Autodesk Inventor part; units mm, degrees
ref_plane "YZ Plane" through (0, 0, 0) normal (1, 0, 0) x (0, 1, 0)
ref_plane "XZ Plane" through (0, 0, 0) normal (0, 1, 0) x (-1, 0, 0)
ref_plane "XY Plane" through (0, 0, 0) normal (0, 0, 1) x (1, 0, 0)
sketch "Sketch1" plane through (0, 0, 0) normal (0, 0, 1) x (1, 0, 0)
  circle A0 centre (0, 0) radius 9.53
  dimension "d0" = 19.06
extrude "Extrusion1" add sketch "Sketch1" against normal blind 20.62
sketch "Sketch2" plane through (0, 0, 0) normal (0, 0, 1) x (1, 0, 0)
  circle A0 centre (0, 0) radius 5.795
  dimension "d3" = 11.59
extrude "Extrusion2" add sketch "Sketch2" along normal blind 6.35
sketch "Sketch3" plane through (0, 0, 6.35) normal (0, 0, 1) x (1, 0, 0)
  circle A0 centre (0, 0) radius 7
  dimension "d6" = 14
extrude "Extrusion3" add sketch "Sketch3" along normal blind 100
sketch "Sketch4" plane through (0, 0, 106.35) normal (0, 0, 1) x (1, 0, 0)
  circle A0 centre (0, 0) radius 7
  circle A1 centre (0, 0) radius 7
  circle A2 centre (0, 0) radius 7
  circle A3 centre (0, 0) radius 5.795
extrude "Extrusion4" add sketch "Sketch4" along normal blind 22.1 contours A3
sketch "Sketch5" plane through (0, 0, 128.45) normal (0, 0, 1) x (1, 0, 0)
  circle A0 centre (0, 0) radius 4.76
  dimension "d11" = 9.52
extrude "Extrusion5" add sketch "Sketch5" along normal blind 3.33
sketch "Sketch6" plane through (0, 0, 131.78) normal (0, 0, 1) x (1, 0, 0)
  circle A0 centre (0, 0) radius 5.795
extrude "Extrusion6" add sketch "Sketch6" along normal blind 6.35
sketch "Sketch7" plane through (0, 0, 0) normal (0, 1, 0) x (-1, 0, 0)
  circle A0 centre (0, -10.31) radius 4.32
  point P0 (0, 0)
  dimension "d16" = 8.64
extrude "Extrusion7" cut sketch "Sketch7" along normal mid plane 40.35
thread "Thread1"
properties part number "parça3"
Input: part model. Units: mm. Frame: model coordinates. A direction names the side the tool comes from. Give positions to 0.01 mm unless a question says otherwise; leave off trailing zeros. Write each loop counter-clockwise with the first axis right and the second up, starting at its lowest first coordinate (ties: lowest second). Pieces come first, ordered by that corner, then holes.
Q1. Section B-B, the plane y = 0. Output: boundary loops of the cut face in (x, z) (3 decimals).
Q2. Pull-direction query (Z, two-part tool) for faces 1 (the face through (5.527, -1.741, 134.911)), 2 (the face through (0, -6, 0)), 3 (the face through (0, 0, 138.13)); classes: pulls with the +Z half, pulls with the -Z half, needs draft (parallel to the pull), parting line crosses it, or undercut.
Q3. Set-up query: faces 4 (the face through (0.936, 0.133, -14.527)), 5 (the face through (-1.032, 4.647, 130.092)), 6 (the face through (6.466, 2.681, 55.65)). Return all of +Z, -Z, +X, -X, +Y, -Y with unobstructed straight access to the full face (end or side cutting, diameter ignored); none if empty.
Q4. First-contact query: P1, Ø2, axis at y = 1, z = 29, coming from the -X side; P2, Ø10, axis at y = -6.5, z = 83, coming from the +X side; P3, Ø10, axis at x = 3, z = 73, coming from the -Y side; P4, Ø7, axis at x = 0, z = -10.31, coming from the +Y side. Flat tips, straight axial feed; report the tip coordinate or a pass-through.
Q5. Section C-C, the plane z = 115.5. Output: boundary loops of the cut face in (x, y) (3 decimals), plus the area to 3 significant figures.
Q6. Material intervals for probe 1 along Z at (x, y) = (0, 5.5); probe 2 along Z at (x, y) = (-0.25, -8); probe 3 along Z at (x, y) = (5.5, -3.5), sorted ascending.
Q7. Section D-D, the plane z = -10.31. Output: boundary loops of the cut face in (x, y), plus the area to 3 significant figures.
Q8. Section A-A, the plane x = 0. Output: boundary loops of the cut face in (y, z) (3 decimals), plus the area to 3 significant figures.
Filled in:
1. outline: (-9.53, -20.62) - (9.53, -20.62) - (9.53, 0) - (5.795, 0) - (5.795, 6.35) - (7, 6.35) - (7, 106.35) - (5.795, 106.35) - (5.795, 128.45) - (4.76, 128.45) - (4.76, 131.78) - (5.795, 131.78) - (5.795, 138.13) - (-5.795, 138.13) - (-5.795, 131.78) - (-4.76, 131.78) - (-4.76, 128.45) - (-5.795, 128.45) - (-5.795, 106.35) - (-7, 106.35) - (-7, 6.35) - (-5.795, 6.35) - (-5.795, 0) - (-9.53, 0) - close; hole circle Ø8.64 at (0, -10.31)
2. face 1: needs draft
2. face 2: undercut
2. face 3: pulls with the +Z half
3. face 4: +Y, -Y
3. face 5: none
3. face 6: +Z
4. P1: stops at x = -7
4. P2: stops at x = 6.84
4. P3: stops at y = -7
4. P4: passes through
5. outline: circle Ø11.59 at (0, 0)
5. area: 106 mm2
6. probe 1: z = -20.62 to -14.63, -5.99 to 128.45, 131.78 to 138.13
6. probe 2: z = -20.62 to -14.62, -6 to 0
6. probe 3: z = -20.62 to 0, 6.35 to 106.35
7. outline: (-4.32, -8.49) - (-4.32, 8.49) arc R9.53 ccw to start; (4.32, -8.49) arc R9.53 ccw to (4.32, 8.49) - close
7. area: 126 mm2
8. outline: (-9.53, -20.62) - (9.53, -20.62) - (9.53, -14.63) - (-9.53, -14.63) - close; (-9.53, -5.99) - (9.53, -5.99) - (9.53, 0) - (5.795, 0) - (5.795, 6.35) - (7, 6.35) - (7, 106.35) - (5.795, 106.35) - (5.795, 128.45) - (4.76, 128.45) - (4.76, 131.78) - (5.795, 131.78) - (5.795, 138.13) - (-5.795, 138.13) - (-5.795, 131.78) - (-4.76, 131.78) - (-4.76, 128.45) - (-5.795, 128.45) - (-5.795, 106.35) - (-7, 106.35) - (-7, 6.35) - (-5.795, 6.35) - (-5.795, 0) - (-9.53, 0) - close
8. area: 2,060 mm2
